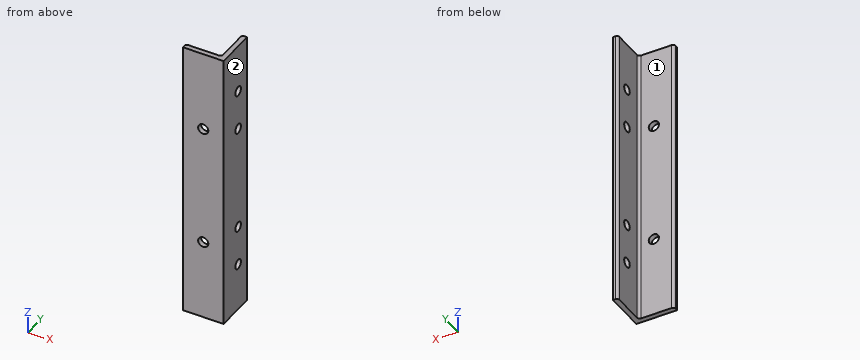
from build123d import *

# Parameters (mm, degrees)
BOSS_EXTRUDE1_DEPTH = 87.698453
SKETCH3_R           = 3.175
CUT_EXTRUDE1_DEPTH  = 93.181715424
SKETCH4_R           = 3
CUT_EXTRUDE2_DEPTH  = 94.968767596


with BuildPart() as part:
    # Sketch2 → Boss-Extrude1 (new, symmetric)
    with BuildSketch(Plane.XY):
        with BuildLine():
            Line((-12.7, 0), (12.7, 0))
            Line((12.7, 0), (12.7, 25.4))
            Line((12.7, 25.4), (11.1125, 25.4))
            ThreePointArc((11.1125, 25.4), (9.989967985, 24.935032015), (9.525, 23.8125))
            Line((9.525, 23.8125), (9.525, 4.7625))
            ThreePointArc((9.525, 4.7625), (9.060032015, 3.639967985), (7.9375, 3.175))
            Line((7.9375, 3.175), (-11.1125, 3.175))
            ThreePointArc((-11.1125, 3.175), (-12.235032015, 2.710032015), (-12.7, 1.5875))
            Line((-12.7, 1.5875), (-12.7, 0))
        make_face()
    extrude(amount=BOSS_EXTRUDE1_DEPTH, both=True)

    # Sketch3 → Cut-Extrude1 (cut, through all)
    with BuildSketch(Plane.XZ):
        with Locations(Location((0, -37.698453, 0), (0, 0, 270))):
            Circle(SKETCH3_R)
        with Locations((0, 37.698453)):
            Circle(SKETCH3_R)
    extrude(amount=-CUT_EXTRUDE1_DEPTH, mode=Mode.SUBTRACT)

    # Sketch4 → Cut-Extrude2 (cut, through all)
    with BuildSketch(Plane.ZY.offset(-9.525)):
        with Locations((-57.698453, 15.647712404)):
            Circle(SKETCH4_R)
        with Locations((-32.698453, 15.647712404)):
            Circle(SKETCH4_R)
        with Locations(Location((57.698453, 15.647712404, 0), (0, 0, 180))):
            Circle(SKETCH4_R)
        with Locations(Location((32.698453, 15.647712404, 0), (0, 0, 180))):
            Circle(SKETCH4_R)
    extrude(amount=-CUT_EXTRUDE2_DEPTH, mode=Mode.SUBTRACT)


solid = part.part
The model under review builds one solid part; all positions refer to its coordinate system, in mm. Face numbers are marked on the shaded views. A direction names the side the tool comes from. Round coordinates to 2 decimals unless told otherwise and drop trailing zeros. Loops run counter-clockwise (first coordinate to the right, second up) from the corner with the lowest first, then second, coordinate; pieces in that order, holes last. Notation, with made-up numbers: (-27, 6) -> (23, 6) arc R27 cw to (23, 35) -> close; hole circle Ø9 at (52.5, 71.25). An arc over 180 degrees is marked (long way). Answer as CSV lines item,"result".
1) Add section A-A on x = 0. Write out the cut boundary in (y, z) (3 decimals).
Geometry results:
outline,"(0, -87.698) -> (3.175, -87.698) -> (3.175, -40.873) -> (0, -40.873) -> close; (0, -34.523) -> (3.175, -34.523) -> (3.175, 34.523) -> (0, 34.523) -> close; (0, 40.873) -> (3.175, 40.873) -> (3.175, 87.698) -> (0, 87.698) -> close"
2) For P1, Ø1.5, axis at y = 15.5, z = 39.5, coming from the -X side (3 decimals); P2, Ø6, axis at x = 3.5, y = 7, coming from the +Z side; P3, Ø5.5, axis at x = 1, z = 35, coming from the +Y side (3 decimals), all flat-tipped, find the tip position at first contact; note any pin that passes through.
Geometry results:
P1,"stops at x = 9.525"
P2,"passes through"
P3,"stops at y = 3.175"
3) Add section C-C on y = 7. Write out the cut boundary in (x, z) (3 decimals), plus the area to 3 significant figures.
Geometry results:
outline,"(9.525, -87.698) -> (12.7, -87.698) -> (12.7, 87.698) -> (9.525, 87.698) -> close"
area,"557 mm²"
4) To check wall thickness, follow line 1 along Z through (x, y) = (-2.75, 2.25); line 2 along X through (y, z) = (13.5, -8) (3 decimals); line 3 along Y through (x, z) = (6, -40) (3 decimals). State the ranges of each line that lie inside material, in increasing order. Write a range as from..to.
Geometry results:
line 1,"z = -87.7..-39.29, -36.11..36.11, 39.29..87.7"
line 2,"x = 9.525..12.7"
line 3,"y = 0..3.175"
5) Tool access review of the marked faces 1 and 2: name each direction out of +Z, -Z, +X, -X, +Y, -Y from which nothing blocks a thin tool from reaching the whole face with its end or side.
Geometry results:
face 1,"+Z, -Z, -X, +Y"
face 2,"+Z, -Z, +X, +Y, -Y"
6) Add section B-B on z = 75.5. Write out the cut boundary in (x, y) (1 decimal).
Geometry results:
outline,"(-12.7, 0) -> (12.7, 0) -> (12.7, 25.4) -> (11.1, 25.4) arc R1.6 ccw to (9.5, 23.8) -> (9.5, 4.8) arc R1.6 cw to (7.9, 3.2) -> (-11.1, 3.2) arc R1.6 ccw to (-12.7, 1.6) -> close"
